```python
from build123d import *

# Parameters (mm, degrees)
SKETCH1_W           = 10
SKETCH1_H           = 10
BOSS_EXTRUDE1_DEPTH = 2.5
BOSS_EXTRUDE2_DEPTH = 2.5
BOSS_EXTRUDE3_DEPTH = 1.5


with BuildPart() as part:
    # Sketch1 → Boss-Extrude1 (new body)
    with BuildSketch(Plane(origin=(0, 0, 0), x_dir=(1, 0, 0), z_dir=(0, 1, 0))):
        Rectangle(SKETCH1_W, SKETCH1_H)
        with BuildLine():
            ThreePointArc((1.617598637, -1.615265837), (3.065, 0), (1.617598637, 1.615265837))
            ThreePointArc((1.617598637, 1.615265837), (1.474163525, 1.620673027), (1.331431871, 1.605489361))
            Line((1.331431871, 1.605489361), (-1.677221968, 1.064808042))
            ThreePointArc((-1.677221968, 1.064808042), (-1.895132853, 0.999347796), (-2.092605578, 0.886322491))
            ThreePointArc((-2.092605578, 0.886322491), (-2.54112078, 0), (-2.092605578, -0.886322491))
            ThreePointArc((-2.092605578, -0.886322491), (-1.895132853, -0.999347796), (-1.677221968, -1.064808042))
            Line((-1.677221968, -1.064808042), (1.331431871, -1.605489361))
            ThreePointArc((1.331431871, -1.605489361), (1.474163525, -1.620673027), (1.617598637, -1.615265837))
        make_face(mode=Mode.SUBTRACT)
    extrude(amount=BOSS_EXTRUDE1_DEPTH)

    # Sketch2 → Boss-Extrude2 (add)
    with BuildSketch(Plane(origin=(0, 0, 0), x_dir=(1, 0, 0), z_dir=(0, 1, 0))):
        Polygon((-2, 6), (-6, 6), (-6, 2), (-5, 2), (-5, 5), (-2, 5), align=None)
        Polygon((2, 6), (2, 5), (5, 5), (5, 2), (6, 2), (6, 6), align=None)
        Polygon((5, -2), (5, -5), (2, -5), (2, -6), (6, -6), (6, -2), align=None)
        Polygon((-6, -2), (-5, -2), (-5, -5), (-2, -5), (-2, -6), (-6, -6), align=None)
    extrude(amount=BOSS_EXTRUDE2_DEPTH)

    # Sketch2_4 → Boss-Extrude3 (add)
    with BuildSketch(Plane(origin=(0, 0, 0), x_dir=(1, 0, 0), z_dir=(0, 1, 0))):
        Polygon((-2, 6), (-6, 6), (-6, 2), (-5, 2), (-5, 5), (-2, 5), align=None)
        Polygon((2, 6), (2, 5), (5, 5), (5, 2), (6, 2), (6, 6), align=None)
        Polygon((5, -2), (5, -5), (2, -5), (2, -6), (6, -6), (6, -2), align=None)
        Polygon((-6, -2), (-5, -2), (-5, -5), (-2, -5), (-2, -6), (-6, -6), align=None)
    extrude(amount=-BOSS_EXTRUDE3_DEPTH)


solid = part.part
```
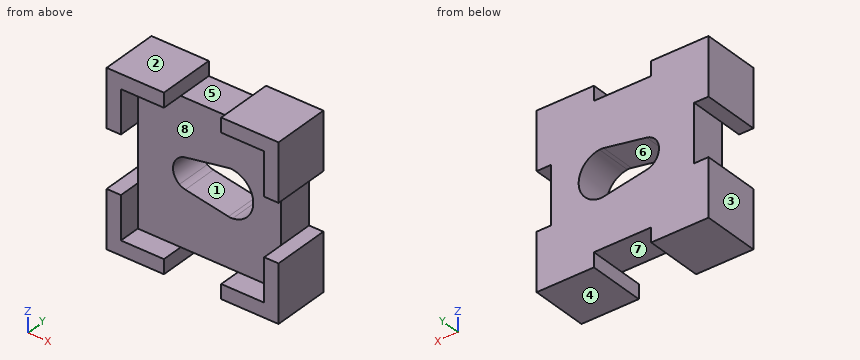
Build history of the part. All positions in model axes, mm. Face numbers are marked on the shaded views. A direction names the side the tool comes from. Give positions to 0.01 mm unless a question says otherwise; leave off trailing zeros. Order: outer loops, then holes, each group sorted by start corner. A loop starts at its lowest first (then second) coordinate and runs counter-clockwise, first axis right, second up. Notation, with made-up numbers: M -0.75,10.5 L 19.25,10.5 A32 cw 19.25,40.5 Z; hole C 67.25,37.5 d10. An arc over 180 degrees is marked long. Write item = value, one per line. Start each with the question number.
(1) Pin check, flat tips, straight feed: pin 1 Ø3 at (x, z) = (1, 0.5) entering from -Y; pin 2 Ø1.2 at (x, y) = (0.5, 1) entering from -Z; pin 3 Ø2 at (y, z) = (1, -0.5) entering from -X. Stop position of each tip, or through.
(2) Probe L1, parallel to Z at x = 5.25, y = 0.65; L2, parallel to X at y = -0.25, z = -3.5; L3, parallel to Y at x = 3.25, z = -2.5. List the from-to ranges inside material, lowest first. Write a range as [from, to].
(3) Two-plate mould, pull along X, no slides. Class the marked faces 1, 2 and 3: released by +X, released by -X, zero draft, split by the parting line, or undercut.
(4) Slice it at D-D on y = -0.7. Write the cut outline in (x, z), plus the area to 3 significant figures.
(5) Which spindle directions (+Z, -Z, +X, -X, +Y, -Y) get a long thin tool onto all of the face, cutting with end or side? Do the marked faces 4, 5, 6, 7 and 8. Say none if no direction does.
(6) Slice it at B-B on z = -3.75. Write the cut outline in (x, y), plus the area to 3 significant figures.
(7) Slice it at A-A on y = 0.8. Write the cut outline in (x, z) (3 decimals), plus the area to 3 significant figures.
(8) Slice it at C-C on x = 0. Write the cut outline in (y, z), plus the area to 3 significant figures.
Responses:
q1.pin_1 = 0
q1.pin_2 = -5
q1.pin_3 = -5
q2.L1 = [-6, -2], [2, 6]
q2.L2 = [-6, -5], [5, 6]
q2.L3 = [0, 2.5]
q3.face_1 = undercut
q3.face_2 = zero draft
q3.face_3 = released by -X
q4.outline = M -6,-6 L -2,-6 L -2,-5 L -5,-5 L -5,-2 L -6,-2 Z; M -6,2 L -5,2 L -5,5 L -2,5 L -2,6 L -6,6 Z; M 2,-6 L 6,-6 L 6,-2 L 5,-2 L 5,-5 L 2,-5 Z; M 2,5 L 5,5 L 5,2 L 6,2 L 6,6 L 2,6 Z
q4.area = 28.0 mm2
q5.face_4 = -Z, +X, -X, +Y, -Y
q5.face_5 = +Z, +Y, -Y
q5.face_6 = +Y, -Y
q5.face_7 = -Z, +Y, -Y
q5.face_8 = -Y
q6.outline = M -6,-1.5 L -5,-1.5 L -5,0 L 5,0 L 5,-1.5 L 6,-1.5 L 6,2.5 L -6,2.5 Z
q6.area = 33.0 mm2
q7.outline = M -6,-6 L -2,-6 L -2,-5 L 2,-5 L 2,-6 L 6,-6 L 6,-2 L 5,-2 L 5,2 L 6,2 L 6,6 L 2,6 L 2,5 L -2,5 L -2,6 L -6,6 L -6,2 L -5,2 L -5,-2 L -6,-2 Z; hole M -2.093,-0.886 A1 ccw -1.677,-1.065 L 1.331,-1.605 A1 ccw 1.618,-1.615 A1.625 ccw 1.618,1.615 A1 ccw 1.331,1.605 L -1.677,1.065 A1 ccw -2.093,0.886 A1.1 ccw Z
q7.area = 114 mm2
q8.outline = M 0,-5 L 2.5,-5 L 2.5,-1.37 L 0,-1.37 Z; M 0,1.37 L 2.5,1.37 L 2.5,5 L 0,5 Z
q8.area = 18.2 mm2
